Read the model definition and answer for the solid it produces. Units are mm, in the model's axes. A direction names the side the tool comes from. Coordinates: 2 decimals unless noted, no trailing zeros. Write each loop counter-clockwise with the first axis right and the second up, starting at its lowest first coordinate (ties: lowest second). Pieces come first, ordered by that corner, then holes. Notation, with made-up numbers: (73, 17) - (119, 17) arc R19 cw to (119, 42) - close; hole circle Ø8 at (14.5, -35.75). An arc over 180 degrees is marked (long way). Return JSON: item names as keys, results as strings.
```python
from build123d import *

# Parameters (mm, degrees)
F0_W     = 88.9
F0_H     = 19.05
F1_DEPTH = 1041.4
F2_W     = 63.5
F2_H     = 19.05
F3_DEPTH = 38.1
F4_W     = 63.5
F4_H     = 19.05
F5_DEPTH = 38.1


with BuildPart() as f1:
    # F0 (on Front) → F1 (new body)
    with BuildSketch(Plane.XZ):
        with Locations((44.45, 9.525)):
            Rectangle(F0_W, F0_H)
    extrude(amount=-F1_DEPTH)

    # F2 (on face) → F3 (join)
    with BuildSketch(Plane.XZ):
        with Locations((44.45, 9.525)):
            Rectangle(F2_W, F2_H)
    extrude(amount=F3_DEPTH)

    # F4 (on face) → F5 (join)
    with BuildSketch(Plane(origin=(0, 1041.4, 0), x_dir=(-1, 0, 0), z_dir=(0, 1, 0))):
        with Locations((-44.45, 9.525)):
            Rectangle(F4_W, F4_H)
    extrude(amount=F5_DEPTH)


solid = f1.part
```
(1) Which of the six approach directions +Z, -Z, +X, -X, +Y, -Y give full straight-line access (tool end or side, diameter ignored) to faces 1 (the face through (12.7, -19, 9)), 2 (the face through (12.7, 1060, 9)), 3 (the face through (76.2, -19, 9)), 4 (the face through (76.2, 1060, 9))?
Answer:
{"face 1": "+Z, -Z, -X, -Y", "face 2": "+Z, -Z, -X, +Y", "face 3": "+Z, -Z, +X, -Y", "face 4": "+Z, -Z, +X, +Y"}
(2) A cutting plane is placed at A-A (z = 4). Determine the outline of the cut face in (x, y), and give its area (3 significant figures).
Answer:
{"outline": "(0, 0) - (12.7, 0) - (12.7, -38.1) - (76.2, -38.1) - (76.2, 0) - (88.9, 0) - (88.9, 1041.4) - (76.2, 1041.4) - (76.2, 1079.5) - (12.7, 1079.5) - (12.7, 1041.4) - (0, 1041.4) - close", "area": "97,400 mm²"}
(3) Flat-ended cylindrical pins translate along their axes: P1, Ø6.5, axis at x = 84, z = 12.5, coming from the -Y side; P2, Ø6.5, axis at x = 85, z = 6, coming from the +Y side. Find the tip coordinate at first contact, or state that the pin passes through.
Answer:
{"P1": "y = 0", "P2": "y = 1041.4"}
(4) A straight line is drawn through the part: line 1 (Y direction, x = 12, z = 10.75). Find the intervals that lie inside material, in ascending order. Write a range as from..to.
Answer:
{"line 1": "0..1041.4"}
